from build123d import *

# Parameters (mm, degrees)
CUT_EXTRUDE1_DEPTH       = 15
CUT_EXTRUDE1_DEPTH_BACK  = 15
SKETCH5_R                = 8
BOSS_EXTRUDE1_DEPTH      = 15
BOSS_EXTRUDE1_DEPTH_BACK = 15
SKETCH6_R                = 5
CUT_EXTRUDE2_DEPTH       = 5
CUT_EXTRUDE2_DEPTH_BACK  = 5
SKETCH7_R                = 5
BOSS_EXTRUDE2_DEPTH      = 5
BOSS_EXTRUDE2_DEPTH_BACK = 5
SKETCH8_R                = 3
SKETCH9_W                = 10
SKETCH9_H                = 5
BOSS_EXTRUDE3_DEPTH      = 10
LPATTERN1_COUNT          = 2
LPATTERN1_PITCH          = 20
BOSS_EXTRUDE4_DEPTH      = 1
BOSS_EXTRUDE4_DEPTH_BACK = 10
SKETCH10_R               = 10
SKETCH11_R               = 7
BOSS_EXTRUDE5_DEPTH      = 2
CUT_EXTRUDE5_DEPTH       = 2
BOSS_EXTRUDE6_DEPTH      = 15
BOSS_EXTRUDE6_DEPTH_BACK = 15
CUT_EXTRUDE6_DEPTH       = 5
CUT_EXTRUDE6_DEPTH_BACK  = 5
SKETCH15_R               = 10
CUT_EXTRUDE7_DEPTH       = 1


with BuildPart() as part:
    # Sketch3 → Revolve2 (revolve)
    with BuildSketch(Plane(origin=(0, 0, 0), x_dir=(0, 0, -1), z_dir=(1, 0, 0)), mode=Mode.PRIVATE) as revolve2_sk:
        with BuildLine():
            Line((50, 0), (40, 0))
            ThreePointArc((40, 0), (28.284271247, -28.284271247), (0, -40))
            Line((0, -40), (0, -50))
            ThreePointArc((0, -50), (35.355339059, -35.355339059), (50, 0))
        make_face()
    revolve(revolve2_sk.sketch.rotate(Axis((0, 0, 0), (0, 1, 0)), 180), axis=Axis((0, 0, 0), (0, 1, 0)))

    # Sketch5 → Cut-Extrude1 (cut, two sides: drawn at the far end of the back side and taken through both)
    with BuildSketch(Plane(origin=(0, 0, 0), x_dir=(0, 0, -1), z_dir=(1, 0, 0)).offset(-CUT_EXTRUDE1_DEPTH_BACK)):
        with Locations((50, 0)):
            Circle(SKETCH5_R)
    extrude(amount=CUT_EXTRUDE1_DEPTH + CUT_EXTRUDE1_DEPTH_BACK, mode=Mode.SUBTRACT)

    # Sketch6 → Boss-Extrude1 (add, two sides: drawn at the far end of the back side and taken through both)
    with BuildSketch(Plane(origin=(0, 0, 0), x_dir=(0, 0, -1), z_dir=(1, 0, 0)).offset(-BOSS_EXTRUDE1_DEPTH_BACK)):
        with Locations(Location((50, 0, 0), (0, 0, 240))):
            Circle(SKETCH6_R)
    extrude(amount=BOSS_EXTRUDE1_DEPTH + BOSS_EXTRUDE1_DEPTH_BACK)

    # Sketch7 → Cut-Extrude2 (cut, two sides: drawn at the far end of the back side and taken through both)
    with BuildSketch(Plane(origin=(0, 0, 0), x_dir=(0, 0, -1), z_dir=(1, 0, 0)).offset(-CUT_EXTRUDE2_DEPTH_BACK)):
        with Locations((50, 0)):
            Circle(SKETCH7_R)
    extrude(amount=CUT_EXTRUDE2_DEPTH + CUT_EXTRUDE2_DEPTH_BACK, mode=Mode.SUBTRACT)

    # Sketch8 → Boss-Extrude2 (add, two sides: drawn at the far end of the back side and taken through both)
    with BuildSketch(Plane(origin=(0, 0, 0), x_dir=(0, 0, -1), z_dir=(1, 0, 0)).offset(-BOSS_EXTRUDE2_DEPTH_BACK)):
        with Locations((50, 0)):
            Circle(SKETCH8_R)
    extrude(amount=BOSS_EXTRUDE2_DEPTH + BOSS_EXTRUDE2_DEPTH_BACK)

    # Sketch9 → Boss-Extrude3 (add)
    with BuildSketch(Plane(origin=(15, 0, 0), x_dir=(0, 0, -1), z_dir=(1, 0, 0))):
        with Locations((45, -2.5)):
            Rectangle(SKETCH9_W, SKETCH9_H)
    boss_extrude3 = extrude(amount=-BOSS_EXTRUDE3_DEPTH)

    # LPattern1: Boss-Extrude3 ×2
    with Locations(*[(-i * LPATTERN1_PITCH, 0, 0) for i in range(1, LPATTERN1_COUNT)]):
        add(boss_extrude3)

    # Sketch10 → Boss-Extrude4 (add, two sides: drawn at the far end of the back side and taken through both)
    with BuildSketch(Plane.XY.offset(50).offset(-BOSS_EXTRUDE4_DEPTH_BACK)):
        Circle(SKETCH10_R)
    extrude(amount=BOSS_EXTRUDE4_DEPTH + BOSS_EXTRUDE4_DEPTH_BACK)

    # Sketch11 → Boss-Extrude5 (add)
    with BuildSketch(Plane.XY.offset(50)):
        Circle(SKETCH11_R)
    extrude(amount=BOSS_EXTRUDE5_DEPTH)

    # Sketch12 → Cut-Extrude5 (cut)
    with BuildSketch(Plane(origin=(0, 0, 0), x_dir=(1, 0, 0), z_dir=(0, 1, 0))):
        with BuildLine():
            Line((-15, 44.542094894), (-15, 40.298883359))
            ThreePointArc((-15, 40.298883359), (-43, 0), (-15, -40.298883359))
            Line((-15, -40.298883359), (-15, -44.542094894))
            ThreePointArc((-15, -44.542094894), (-46.999981038, 0), (-15, 44.542094894))
        make_face()
        with BuildLine():
            Line((15, 44.542094894), (15, 40.298883359))
            ThreePointArc((15, 40.298883359), (43, 0), (15, -40.298883359))
            Line((15, -40.298883359), (15, -44.542094894))
            ThreePointArc((15, -44.542094894), (46.999981038, 0), (15, 44.542094894))
        make_face()
    extrude(amount=-CUT_EXTRUDE5_DEPTH, mode=Mode.SUBTRACT)

    # Sketch13 → Boss-Extrude6 (add, two sides: drawn at the far end of the back side and taken through both)
    with BuildSketch(Plane(origin=(0, 0, 0), x_dir=(0, 0, -1), z_dir=(1, 0, 0)).offset(-BOSS_EXTRUDE6_DEPTH_BACK)):
        with BuildLine():
            Line((49.749371855, -5), (40, -5))
            Line((40, -5), (40, -8))
            Line((40, -8), (49.355850717, -8))
            ThreePointArc((49.355850717, -8), (49.57530923, -6.502977374), (49.749371855, -5))
        make_face()
    extrude(amount=BOSS_EXTRUDE6_DEPTH + BOSS_EXTRUDE6_DEPTH_BACK)

    # Sketch14 → Cut-Extrude6 (cut, two sides: drawn at the far end of the back side and taken through both)
    with BuildSketch(Plane(origin=(0, 0, 0), x_dir=(0, 0, -1), z_dir=(1, 0, 0)).offset(-CUT_EXTRUDE6_DEPTH_BACK)):
        with BuildLine():
            Line((49.749371855, -5), (40, -5))
            Line((40, -5), (40, -8))
            Line((40, -8), (49.355850717, -8))
            ThreePointArc((49.355850717, -8), (49.57530923, -6.502977374), (49.749371855, -5))
        make_face()
    extrude(amount=CUT_EXTRUDE6_DEPTH + CUT_EXTRUDE6_DEPTH_BACK, mode=Mode.SUBTRACT)

    # Sketch15 → Cut-Extrude7 (cut)
    with BuildSketch(Plane(origin=(0, -50, 0), x_dir=(1, 0, 0), z_dir=(0, 1, 0))):
        Circle(SKETCH15_R)
    extrude(amount=CUT_EXTRUDE7_DEPTH, mode=Mode.SUBTRACT)


solid = part.part
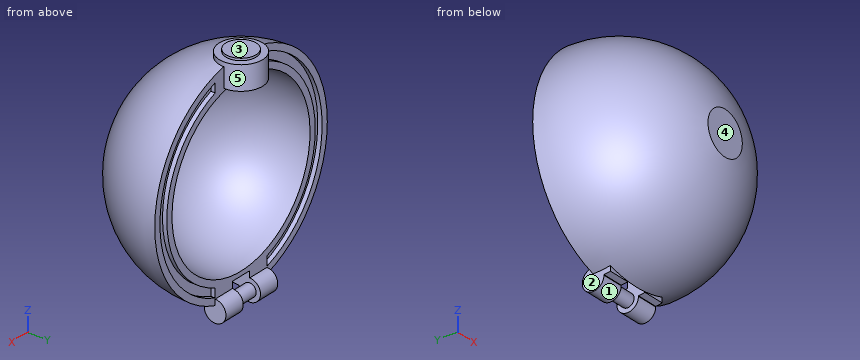
The listing builds one solid part. Answer for the finished solid, in the listing's coordinates (mm). Face numbers are marked on the shaded views. A direction names the side the tool comes from. Coordinates: 2 decimals unless noted, no trailing zeros. Write each loop counter-clockwise with the first axis right and the second up, starting at its lowest first coordinate (ties: lowest second). Pieces come first, ordered by that corner, then holes. Notation, with made-up numbers: (-21, 21) -> (32, 21) arc R10 ccw to (32, 40) -> close; hole circle Ø7 at (64.25, 86.5). An arc over 180 degrees is marked (long way). One line per question, with ' | ' between items.
1. Section B-B (z = 33.5) is taken. Determine the outline of the cut face in (x, y).
Verdict:
outline: (-37.12, 0) arc R37.12 ccw to (37.12, 0) -> (32.97, 0) -> (32.97, -2) -> (26.96, -2) -> (26.96, 0) -> (21.86, 0) arc R21.86 cw to (-21.86, 0) -> (-26.96, 0) -> (-26.96, -2) -> (-32.97, -2) -> (-32.97, 0) -> close
2. Given pin 1 Ø12 at (x, y) = (3, -35) entering from -Z; pin 2 Ø2 at (x, y) = (-29.5, -27) entering from -Z; pin 3 Ø6 at (y, z) = (-1.5, -7.5) entering from +X, each flat-ended and moving along its own axis, determine where each tip first touches the part or whether it passes through.
Verdict:
pin 1: stops at z = -40.64 | pin 2: stops at z = -31.3 | pin 3: stops at x = 49.78
3. Section C-C (x = -30.5) is taken. Determine the outline of the cut face in (y, z), and give its area (3 significant figures).
Verdict:
outline: (-2, -35.76) -> (-2, -30.31) -> (0, -30.31) -> (0, -25.88) arc R25.88 cw to (0, 25.88) -> (0, 30.31) -> (-2, 30.31) -> (-2, 35.76) -> (0, 35.76) -> (0, 39.62) arc R39.62 ccw to (0, -39.62) -> (0, -35.76) -> close | area: 1,390 mm^2
4. Which of the six approach directions +Z, -Z, +X, -X, +Y, -Y give full straight-line access (tool end or side, diameter ignored) to the marked faces 4 and 5?
Verdict:
face 4: +Z, -Z, +X, -X, -Y | face 5: +Z
5. For a pull along Z with two mould halves and no side action, classify the marked faces 1, 2 and 3 as released by +Z, released by -Z, zero draft, split by the parting line, or undercut.
Verdict:
face 1: undercut | face 2: zero draft | face 3: released by +Z
6. Straight lines are drawn through the part: line 1 (X direction, y = -4.5, z = 20); line 2 (X direction, y = -7.5, z = 17); line 3 (Z direction, x = 6.5, y = -7). For each, find the intervals that lie inside material, in ascending order.
Verdict:
line 1: x = -45.6 to -34.35, 34.35 to 45.6 | line 2: x = -46.42 to -35.42, 35.42 to 46.42 | line 3: z = -49.51 to -38.84, 38.84 to 51
7. Section D-D (y = -17) is taken. Determine the outline of the cut face in (x, z), and give its area (3 significant figures).
Verdict:
outline: circle Ø94.04 at (0, 0); hole circle Ø72.42 at (0, 0) | area: 2,830 mm^2
